```python
from build123d import *

# Parameters (mm, degrees)
BOSS_EXTRU_1_DEPTH      = 7
ENL_V_START             = -4
ENL_V_MAT_EXTRU_1_DEPTH = 22.382453919
D_GAGEMENT_M21_D        = 2.4
EMPREINTE1_OUTLINE_R    = 1.2
EMPREINTE1_DEPTH        = 2


# Read off the part's stored shape, not the designer's step: Empreinte1
with BuildPart() as part:
    # Esquisse1 → Boss.-Extru.1 (new, symmetric)
    with BuildSketch(Plane.XY):
        Polygon((4, 0), (4, 13.229473419), (7.5, 11.208747477), (7.5, 3.5), (17, 3.5), (17, 5.72391992), (20.5, 3.703193978), (20.5, 0), align=None)
    extrude(amount=BOSS_EXTRU_1_DEPTH, both=True)

    # Esquisse2 → Enlèv. mat.-Extru.1 (cut, through all)
    with BuildSketch(Plane.XY.offset(ENL_V_START)):
        Polygon((4, 13.229473419), (4, 11.497422612), (7.5, 9.47669667), (7.5, 11.208747477), align=None)
        Polygon((17, 5.72391992), (17, 3.991869112), (20.5, 1.97114317), (20.5, 3.703193978), align=None)
    enl_v_mat_extru_1 = extrude(amount=-ENL_V_MAT_EXTRU_1_DEPTH, mode=Mode.SUBTRACT)

    # Symétrie1: Enlèv. mat.-Extru.1 across plane
    add(enl_v_mat_extru_1.mirror(Plane.XY), mode=Mode.SUBTRACT)

    # Dégagement M21 (through all)
    with Locations(Plane(origin=(0, 0, 0), x_dir=(-1, 0, 0), z_dir=(0, -1, 0))):
        with Locations((-15, 0)):
            Hole(D_GAGEMENT_M21_D / 2)

    # Empreinte1 outline → Empreinte1 (cut)
    with BuildSketch(Plane(origin=(0, 0, 0), x_dir=(1, 0, 0), z_dir=(0, 1, 0))):
        with BuildLine():
            Line((4, -3.115617227), (15.2, -1.989974874))
            ThreePointArc((15.2, -1.989974874), (17, 0), (15.2, 1.989974874))
            Line((15.2, 1.989974874), (4, 3.115617227))
            Line((4, 3.115617227), (4, -3.115617227))
        make_face()
        with Locations((15, 0)):
            Circle(EMPREINTE1_OUTLINE_R, mode=Mode.SUBTRACT)
    extrude(amount=EMPREINTE1_DEPTH, mode=Mode.SUBTRACT)


solid = part.part
```
Geometry: final body of the model. Coordinates: model frame, mm. A direction names the side the tool comes from. Round coordinates to 2 decimals unless told otherwise and drop trailing zeros. Write each loop counter-clockwise with the first axis right and the second up, starting at its lowest first coordinate (ties: lowest second). Pieces come first, ordered by that corner, then holes. Notation, with made-up numbers: M 29.5,68.5 L 71.5,68.5 A16 cw 71.5,74.5 Z; hole C -18.75,32.5 d4. An arc over 180 degrees is marked long. Answer in a Markdown table with one row per item. Add a question column.
(1) Ray query, L1, parallel to Z at x = 15, y = 3.1; L2, parallel to X at y = 3.15, z = 0; L3, parallel to Y at x = 8.5, z = -0.5. Return the intervals inside material, ascending.
(2) Cut plane C-C, the plane x = 18.5. Return the cut outline in (y, z).
(3) Cut plane D-D, the plane y = 4.5. Return the cut outline in (x, z), then the cut area to 3 significant figures.
(4) Draft query along Z for faces 6 (the face through (17, 1, 0)), 7 (the face through (19, 4, -4)), 8 (the face through (12, 0, 3)). Return one class per face: pulls with the +Z half, pulls with the -Z half, needs draft (parallel to the pull), parting line crosses it, or undercut.
(5) Contact query for flat-ended pins moving along their axis: pin 1 (3 mm diameter, centred on x = 17, z = -1.5, fed in from +Y); pin 2 (1.4 mm diameter, centred on x = 15, z = 0, fed in from -Y); pin 3 (1 mm diameter, centred on x = 5.5, y = 11.5, fed in from -Z); pin 4 (6 mm diameter, centred on y = 8.5, z = -1.5, fed in from +X). Output: stop coordinate, or through.
(6) Reachability of faces 1 (the face through (18.726, 4.728, 0.056)), 2 (the face through (5.73, 10.5, 5.48)), 3 (the face through (17, 4, 0)), 4 (the face through (9.678, 0.986, -2.545)), 5 (the face through (18.726, 2.996, -5.479)) from +Z, -Z, +X, -X, +Y, -Y: full face, straight path, thin tool, end or side. Return the list, or none.
(7) Cut plane B-B, the plane z = 0. Return the cut outline in (x, y).
(8) Cut plane A-A, the plane y = 1. Return the cut outline in (x, z).
Established:
| question | item | result |
|---|---|---|
| 1 | L1 | -7 to -1.2, 1.2 to 7 |
| 1 | L2 | 4 to 13.8, 16.2 to 20.5 |
| 1 | L3 | 2 to 3.5 |
| 2 | outline | M 0,-7 L 3.13,-7 L 3.13,-4 L 4.86,-4 L 4.86,4 L 3.13,4 L 3.13,7 L 0,7 Z |
| 3 | outline | M 4,-7 L 7.5,-7 L 7.5,7 L 4,7 Z; M 17,-4 L 19.12,-4 L 19.12,4 L 17,4 Z |
| 3 | area | 66.0 mm² |
| 4 | face 6 | undercut |
| 4 | face 7 | pulls with the -Z half |
| 4 | face 8 | needs draft |
| 5 | pin 1 | y = 5.72 |
| 5 | pin 2 | through |
| 5 | pin 3 | z = -4 |
| 5 | pin 4 | x = 17.39 |
| 6 | face 1 | +Z, -Z, +X, +Y |
| 6 | face 2 | +Z, +X, +Y |
| 6 | face 3 | +Z, -Z, +Y |
| 6 | face 4 | -X, -Y |
| 6 | face 5 | -Z, +X, +Y |
| 7 | outline | M 4,2 L 13.8,2 L 13.8,3.5 L 7.5,3.5 L 7.5,11.21 L 4,13.23 Z; M 16.2,2 L 17,2 L 17,0 L 20.5,0 L 20.5,3.7 L 17,5.72 L 17,3.5 L 16.2,3.5 Z |
| 8 | outline | M 4,-7 L 20.5,-7 L 20.5,7 L 4,7 L 4,3.12 L 15.2,1.99 A2 cw 15.2,-1.99 L 4,-3.12 Z |
